Work out the finished part from the listing and answer in its coordinate system (mm). Face numbers are marked on the shaded views. A direction names the side the tool comes from. Coordinates: 2 decimals unless noted, no trailing zeros. Write each loop counter-clockwise with the first axis right and the second up, starting at its lowest first coordinate (ties: lowest second). Pieces come first, ordered by that corner, then holes. Notation, with made-up numbers: (52, 64.25) - (63, 64.25) arc R16 ccw to (63, 91.25) - close; hole circle Ø2 at (-5.5, 74). An arc over 180 degrees is marked (long way). Use a Markdown table: item, result. Add a question column.
(1) The part is cut by section C-C, the plane z = -8.5. Give the vertices of the cut face in (x, y).
(2) Given pin 1 Ø0.5 at (y, z) = (-1.5, -18) entering from +X; pin 2 Ø2 at (y, z) = (16.5, 19.5) entering from -X; pin 3 Ø1.9 at (y, z) = (-1, -17) entering from -X, each flat-ended and moving along its own axis, determine where each tip first touches the part or whether it passes through.
(3) The part is cut by section B-B, the plane z = 5. Give the vertices of the cut face in (x, y), then the cut area to 3 significant figures.
(4) Find the intervals of material crossed by line 1 (X direction, y = -0.5, z = 5); line 2 (Y direction, x = 2, z = -1.5); line 3 (Z direction, x = 4, y = 4), in increasing order. Write a range as from..to.
(5) A tool of negligible diameter and unlimited length cuts with its end or side. For the marked faces 4 and 5, from which of +Z, -Z, +X, -X, +Y, -Y can it reach the whole face along a straight path? Write none if from no direction.
(6) For a pull along Z with two mould halves and no side action, classify the marked faces 1, 2 and 3 as released by +Z, released by -Z, zero draft, split by the parting line, or undercut.
(7) The part is cut by section A-A, the plane y = 12. Give the vertices of the cut face in (x, z).
from build123d import *

# Parameters (mm, degrees)
BRIDA_BASE1_DEPTH               = 2
PLIEGUE_START                   = -10.5
PLIEGUE_CROQUIZADO2_DEPTH       = 21
PLIEGUE_CROQUIZADO2_2_OUTLINE_W = 36.429203673
PLIEGUE_CROQUIZADO2_2_OUTLINE_H = 2
PLIEGUE_CROQUIZADO2_2_DEPTH     = 21
CROQUIS9_R                      = 1.5
CORTAR_EXTRUIR1_DEPTH           = 51.180268834
CORTAR_EXTRUIR2_DEPTH           = 62.824160975
CORTAR_EXTRUIR2_DEPTH_BACK      = 62.824160975
CROQUIS10_R                     = 1.25
CROQUIS10_R_2                   = 3
REDONDEO3_R                     = 3
REDONDEO4_R                     = 0.5


# Read off the part's stored shape, not the designer's step: Pliegue croquizado2
# Sheet-metal steps are written as plain solids
with BuildPart() as part:
    # Croquis1 → Brida base1 (new body)
    with BuildSketch(Plane(origin=(0, 0, 0), x_dir=(1, 0, 0), z_dir=(0, 1, 0))):
        with BuildLine():
            Line((10.5, 18.85), (20.023174074, 18.85))
            ThreePointArc((20.023174074, 18.85), (27.5, 0), (20.023174074, -18.85))
            Line((20.023174074, -18.85), (10.5, -18.85))
            Line((10.5, -18.85), (10.5, -56.85))
            Line((10.5, -56.85), (-10.5, -56.85))
            Line((-10.5, -56.85), (-10.5, -18.85))
            Line((-10.5, -18.85), (-20.023174074, -18.85))
            ThreePointArc((-20.023174074, -18.85), (-27.5, 0), (-20.023174074, 18.85))
            Line((-20.023174074, 18.85), (-10.5, 18.85))
            Line((-10.5, 18.85), (-10.5, 56.85))
            Line((-10.5, 56.85), (10.5, 56.85))
            Line((10.5, 56.85), (10.5, 18.85))
        make_face()
    extrude(amount=-BRIDA_BASE1_DEPTH)

    # Pliegue croquizado2 outline → Pliegue croquizado2 (cut)
    with BuildSketch(Plane.YZ.offset(PLIEGUE_START)):
        with BuildLine():
            Line((0, -56.85), (0, -20.85))
            ThreePointArc((0, -20.85), (-1.414213562, -20.264213562), (-2, -18.85))
            Line((-2, -18.85), (-2, -56.85))
            Line((-2, -56.85), (0, -56.85))
        make_face()
        with BuildLine():
            Line((-2, 56.85), (-2, 18.85))
            ThreePointArc((-2, 18.85), (-1.414213562, 20.264213562), (0, 20.85))
            Line((0, 20.85), (0, 56.85))
            Line((0, 56.85), (-2, 56.85))
        make_face()
    extrude(amount=PLIEGUE_CROQUIZADO2_DEPTH, mode=Mode.SUBTRACT)

    # Pliegue croquizado2 2 outline → Pliegue croquizado2 2 (add)
    with BuildSketch(Plane.YZ.offset(PLIEGUE_START)):
        with Locations((18.214601837, -19.85)):
            Rectangle(PLIEGUE_CROQUIZADO2_2_OUTLINE_W, PLIEGUE_CROQUIZADO2_2_OUTLINE_H)
        with Locations((18.214601837, 19.85)):
            Rectangle(PLIEGUE_CROQUIZADO2_2_OUTLINE_W, PLIEGUE_CROQUIZADO2_2_OUTLINE_H)
    extrude(amount=PLIEGUE_CROQUIZADO2_2_DEPTH)

    # Croquis9 → Cortar-Extruir1 (cut, through all)
    with BuildSketch(Plane(origin=(0, 0, 0), x_dir=(1, 0, 0), z_dir=(0, 1, 0))):
        with Locations(Location((-7.5, 5, 0), (0, 0, 270))):
            Circle(CROQUIS9_R)
        with Locations(Location((-7.5, -5, 0), (0, 0, 270))):
            Circle(CROQUIS9_R)
        with Locations(Location((7.5, -5, 0), (0, 0, 270))):
            Circle(CROQUIS9_R)
        with Locations(Location((7.5, 5, 0), (0, 0, 270))):
            Circle(CROQUIS9_R)
        with BuildLine():
            Line((-18.5815, 16.5815), (-18.5815, 18.85))
            Line((-18.5815, 18.85), (-14.5815, 18.85))
            Line((-14.5815, 18.85), (-14.5815, 16.5815))
            ThreePointArc((-14.5815, 16.5815), (-16.5815, 14.5815), (-18.5815, 16.5815))
        make_face()
        with BuildLine():
            Line((14.5815, 18.85), (18.5815, 18.85))
            Line((18.5815, 18.85), (18.5815, 16.5815))
            ThreePointArc((18.5815, 16.5815), (16.5815, 14.5815), (14.5815, 16.5815))
            Line((14.5815, 16.5815), (14.5815, 18.85))
        make_face()
        with BuildLine():
            Line((14.5815, -18.85), (18.5815, -18.85))
            Line((18.5815, -18.85), (18.5815, -16.5815))
            ThreePointArc((18.5815, -16.5815), (16.5815, -14.5815), (14.5815, -16.5815))
            Line((14.5815, -16.5815), (14.5815, -18.85))
        make_face()
        with BuildLine():
            Line((-18.5815, -16.5815), (-18.5815, -18.85))
            Line((-18.5815, -18.85), (-14.5815, -18.85))
            Line((-14.5815, -18.85), (-14.5815, -16.5815))
            ThreePointArc((-14.5815, -16.5815), (-16.5815, -14.5815), (-18.5815, -16.5815))
        make_face()
    extrude(amount=-CORTAR_EXTRUIR1_DEPTH, mode=Mode.SUBTRACT)

    # Croquis10 → Cortar-Extruir2 (cut, two sides: drawn at the far end of the back side and taken through both)
    with BuildSketch(Plane.XY.offset(20.85).offset(-CORTAR_EXTRUIR2_DEPTH_BACK)):
        with BuildLine():
            ThreePointArc((-10.5, 25.929203673), (-7.424621199, 33.353824879), (8e-09, 36.429203673))
            Line((8e-09, 36.429203673), (-10.5, 36.429203673))
            Line((-10.5, 36.429203673), (-10.5, 25.929203673))
        make_face()
        with BuildLine():
            ThreePointArc((8e-09, 36.429203673), (7.424621205, 33.353824873), (10.5, 25.929203673))
            Line((10.5, 25.929203673), (10.5, 36.429203673))
            Line((10.5, 36.429203673), (8e-09, 36.429203673))
        make_face()
        with Locations(Location((0, 18.579203673, 0), (0, 0, 90))):
            Circle(CROQUIS10_R)
        with Locations(Location((0, 25.929203673, 0), (0, 0, 90))):
            Circle(CROQUIS10_R_2)
        with Locations(Location((7.35, 25.929203673, 0), (0, 0, 90))):
            Circle(CROQUIS10_R)
        with Locations(Location((0, 33.279203673, 0), (0, 0, 90))):
            Circle(CROQUIS10_R)
        with Locations(Location((-7.35, 25.929203673, 0), (0, 0, 90))):
            Circle(CROQUIS10_R)
    extrude(amount=CORTAR_EXTRUIR2_DEPTH + CORTAR_EXTRUIR2_DEPTH_BACK, mode=Mode.SUBTRACT)

    # Redondeo3
    redondeo3_edges = [part.edges().sort_by_distance(p)[0] for p in [
        (20.023174074, -1, -18.85),
        (20.023174074, -1, 18.85),
        (-20.023174074, -1, 18.85),
        (-20.023174074, -1, -18.85),
    ]]
    fillet(redondeo3_edges, radius=REDONDEO3_R)

    # Redondeo4
    redondeo4_edges = [part.edges().sort_by_distance(p)[0] for p in [
        (18.5815, -1, 18.85),
        (14.5815, -1, 18.85),
        (18.5815, -1, -18.85),
        (14.5815, -1, -18.85),
        (-18.5815, -1, 18.85),
        (-14.5815, -1, 18.85),
        (-18.5815, -1, -18.85),
        (-14.5815, -1, -18.85),
    ]]
    fillet(redondeo4_edges, radius=REDONDEO4_R)


solid = part.part
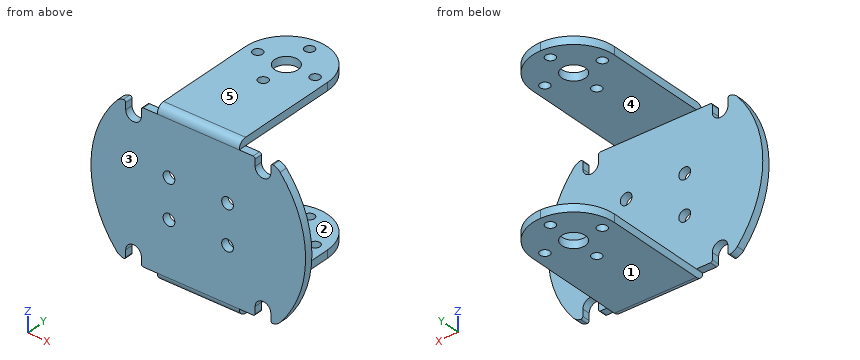
Model answer:
| question | item | result |
|---|---|---|
| 1 | outline | (-26.15, -2) - (26.15, -2) - (26.15, 0) - (-26.15, 0) - close |
| 2 | pin 1 | x = 21 |
| 2 | pin 2 | x = -10.5 |
| 2 | pin 3 | x = -22.33 |
| 3 | outline | (-27.04, -2) - (-9, -2) - (-9, 0) - (-27.04, 0) - close; (-6, -2) - (6, -2) - (6, 0) - (-6, 0) - close; (9, -2) - (27.04, -2) - (27.04, 0) - (9, 0) - close |
| 3 | area | 96.2 mm^2 |
| 4 | line 1 | -27.04..-9, -6..6, 9..27.04 |
| 4 | line 2 | -2..0 |
| 4 | line 3 | -20.85..-18.85, 18.85..20.85 |
| 5 | face 4 | +X, -X, +Y |
| 5 | face 5 | +Z, +X, -X, +Y, -Y |
| 6 | face 1 | released by -Z |
| 6 | face 2 | undercut |
| 6 | face 3 | zero draft |
| 7 | outline | (-10.5, -20.85) - (10.5, -20.85) - (10.5, -18.85) - (-10.5, -18.85) - close; (-10.5, 18.85) - (10.5, 18.85) - (10.5, 20.85) - (-10.5, 20.85) - close |
